```python
from build123d import *

# Parameters (mm, degrees)
SKETCH1_W           = 50
SKETCH1_H           = 50
SKETCH1_R           = 0.5
BOSS_EXTRUDE1_DEPTH = 0.4
BOSS_EXTRUDE2_DEPTH = 0.381


with BuildPart() as part:
    # Sketch1 → Boss-Extrude1 (new body)
    with BuildSketch(Plane(origin=(0, 0, 0), x_dir=(1, 0, 0), z_dir=(0, 1, 0))):
        Rectangle(SKETCH1_W, SKETCH1_H)
        with Locations(Location((0, 0, 0), (0, 0, 270))):
            Circle(SKETCH1_R, mode=Mode.SUBTRACT)
    extrude(amount=BOSS_EXTRUDE1_DEPTH)

    # Sketch3 → Boss-Extrude2 (add)
    with BuildSketch(Plane(origin=(0, 0, 0), x_dir=(1, 0, 0), z_dir=(0, 1, 0))):
        with BuildLine():
            ThreePointArc((38, 0), (-22.60331834, 30.546521897), (-11.11, -36.339618875))
            Line((-11.11, -36.339618875), (11.11, -36.339618875))
            ThreePointArc((11.11, -36.339618875), (30.546521897, -22.60331834), (38, 0))
        make_face()
    extrude(amount=BOSS_EXTRUDE2_DEPTH)


solid = part.part
```
Geometry check sheet. Reference: the model listing, model coordinates, mm. Coordinates: 2 decimals unless noted, no trailing zeros. Order: outer loops, then holes, each group sorted by start corner. A loop starts at its lowest first (then second) coordinate and runs counter-clockwise, first axis right, second up.
Item 1: Section check D-D (z = 30). Enter the section's corners in (x, y), plus the area to 3 significant figures.
Item 2: Scan lines: line 1 along Y through (x, z) = (-7.5, -25.5); line 2 along Z through (x, y) = (-1, 0.1); line 3 along X through (y, z) = (0.3, -14). Record each from-to range of solid material in increasing order.
Item 3: Section check C-C (y = 0.1). Enter the section's corners in (x, z).
Check sheet entries:
1. outline: (-23.32, 0) - (23.32, 0) - (23.32, 0.38) - (-23.32, 0.38) - close
1. area: 17.8 mm2
2. line 1: y = 0 to 0.38
2. line 2: z = -37.99 to 36.34
2. line 3: x = -35.33 to 35.33
3. outline: (-11.11, 36.34) arc R38 ccw (long way) to (11.11, 36.34) - close
